from build123d import *

# Parameters (mm, degrees)
DODANIE_WYCI_GNI_CIE1_DEPTH = 180
WYTNIJ_WYCI_GNI_CIE1_DEPTH  = 181.958558792
SZKIC3_R                    = 2.1
DODANIE_WYCI_GNI_CIE2_DEPTH = 3
SFAZOWANIE1_DEPTH           = 3


with BuildPart() as part:
    # Szkic1 → Dodanie-wyciągnięcie1 (new body)
    with BuildSketch(Plane.XY):
        Polygon((0, 0), (10, 0), (10, 3), (3, 3), (3, 6), (11, 6), (11, 7), (7, 15), (6, 15), (6, 9), (3, 9), (3, 15), (0, 15), align=None)
    extrude(amount=DODANIE_WYCI_GNI_CIE1_DEPTH)

    # Szkic2 → Wytnij-wyciągnięcie1 (cut, through all)
    with BuildSketch(Plane(origin=(0, 15, 0), x_dir=(1, 0, 0), z_dir=(0, 1, 0))):
        Polygon((0, -180), (11, -180), (0, -169), align=None)
    extrude(amount=-WYTNIJ_WYCI_GNI_CIE1_DEPTH, mode=Mode.SUBTRACT)

    # Szkic3 → Dodanie-wyciągnięcie2 (add)
    # profile 1 of 2: a face of its own
    with BuildSketch(Plane.ZY):
        with BuildLine():
            Line((25, 20), (25, 11.336506418))
            Line((25, 11.336506418), (35, 11.336506418))
            Line((35, 11.336506418), (35, 20))
            ThreePointArc((35, 20), (30, 25), (25, 20))
        make_face()
        with Locations((30, 20)):
            Circle(SZKIC3_R, mode=Mode.SUBTRACT)
    # profile 2 of 2: a face of its own
    with BuildSketch(Plane.ZY):
        with BuildLine():
            Line((134, 20), (134, 11.336506418))
            Line((134, 11.336506418), (144, 11.336506418))
            Line((144, 11.336506418), (144, 20))
            ThreePointArc((144, 20), (139, 25), (134, 20))
        make_face()
        with Locations((139, 20)):
            Circle(SZKIC3_R, mode=Mode.SUBTRACT)
    extrude(amount=-DODANIE_WYCI_GNI_CIE2_DEPTH)

    # Sfazowanie1: read off the stored shape, not the designer's step
    # Sfazowanie1 outline → Sfazowanie1 (add)
    with BuildSketch(Plane.YZ):
        with BuildLine():
            Line((15, 134), (15, 124.857864376))
            Line((15, 124.857864376), (21.666666667, 134.285954792))
            ThreePointArc((21.666666667, 134.285954792), (20.845509894, 134.072007202), (20, 134))
            Line((20, 134), (15, 134))
        make_face()
        with BuildLine():
            Line((15, 15.857864376), (21.666666667, 25.285954792))
            ThreePointArc((21.666666667, 25.285954792), (20.845509894, 25.072007202), (20, 25))
            Line((20, 25), (15, 25))
            Line((15, 25), (15, 15.857864376))
        make_face()
        with BuildLine():
            Line((21.666666667, 34.714045208), (15, 44.142135624))
            Line((15, 44.142135624), (15, 35))
            Line((15, 35), (20, 35))
            ThreePointArc((20, 35), (20.845509894, 34.927992798), (21.666666667, 34.714045208))
        make_face()
        with BuildLine():
            ThreePointArc((20, 144), (20.845509894, 143.927992798), (21.666666667, 143.714045208))
            Line((21.666666667, 143.714045208), (15, 153.142135624))
            Line((15, 153.142135624), (15, 144))
            Line((15, 144), (20, 144))
        make_face()
    extrude(amount=SFAZOWANIE1_DEPTH)


solid = part.part
The model under review builds one solid part; all positions refer to its coordinate system, in mm. A direction names the side the tool comes from. Give positions to 0.01 mm unless a question says otherwise; leave off trailing zeros. Write each loop counter-clockwise with the first axis right and the second up, starting at its lowest first coordinate (ties: lowest second). Pieces come first, ordered by that corner, then holes.
1. Wall thickness on L1, parallel to Y at x = 5, z = 102; L2, parallel to Y at x = 1.75, z = 30; L3, parallel to X at y = 9.5, z = 31.5: over which ranges is each line inside the solid? List them lowest first.
2. Tool access review of faces 1 (the flat face through (3, 4, 85)), 2 (the flat face through (1.48, 18.38, 39.36)), 3 (the flat face through (6, 12, 86)), 4 (the flat face through (2, 15, 8)), 5 (the flat face through (10, 1, 88)): name each direction out of +Z, -Z, +X, -X, +Y, -Y from which nothing blocks a thin tool from reaching the whole face with its end or side.
3. For P1, Ø1.5, axis at y = 4, z = 78, coming from the +X side; P2, Ø1.5, axis at y = 18, z = 124.5, coming from the -X side; P3, Ø2.5, axis at x = 1, z = 92, coming from the +Y side; P4, Ø8, axis at y = 14, z = 50.5, coming from the +X side, all flat-tipped, find the tip position at first contact; note any pin that passes through.
4. Draft analysis for pull direction Z (two halves, no side actions). For faces 6 (the flat face through (0, 10, 86)), 7 (the flat face through (1.48, 18.38, 148.36)), 8 (the flat face through (4, 8, 0)), 9 (the flat face through (2, 15, 84)), state which applies: +Z half, -Z half, draft (parallel to the pull), parting line (faces both ways), or undercut.
5. Add section C-C, the plane z = 101.5. Write out the cut boundary in (x, y), plus the area to 3 significant figures.
6. Add section A-A, the plane z = 139. Write out the cut boundary in (x, y), plus the area to 3 significant figures.
7. Add section B-B, the plane y = 20. Write out the cut boundary in (x, z).
8. Add section D-D, the plane y = 4.5. Write out the cut boundary in (x, z).
Worked answers:
1. L1: y = 0 to 3, 6 to 9
1. L2: y = 0 to 17.9, 22.1 to 25
1. L3: x = 0 to 3, 6 to 9.75
2. face 1: +Z, -Z, +X
2. face 2: +X, -X, +Y
2. face 3: +Z, -Z, +Y
2. face 4: -Z, +X, -X, +Y
2. face 5: +Z, -Z, +X, -Y
3. P1: stops at x = 3
3. P2: passes through
3. P3: stops at y = 15
3. P4: stops at x = 9.5
4. face 6: draft
4. face 7: +Z half
4. face 8: -Z half
4. face 9: undercut
5. outline: (0, 0) - (10, 0) - (10, 3) - (3, 3) - (3, 6) - (11, 6) - (11, 7) - (7, 15) - (6, 15) - (6, 9) - (3, 9) - (3, 15) - (0, 15) - close
5. area: 104 mm2
6. outline: (0, 0) - (10, 0) - (10, 3) - (3, 3) - (3, 6) - (11, 6) - (11, 7) - (7, 15) - (6, 15) - (6, 9) - (3, 9) - (3, 17.9) - (0, 17.9) - close; (0, 22.1) - (3, 22.1) - (3, 25) - (0, 25) - close
6. area: 121 mm2
7. outline: (0, 22.93) - (3, 22.93) - (3, 27.9) - (0, 27.9) - close; (0, 32.1) - (3, 32.1) - (3, 37.07) - (0, 37.07) - close; (0, 131.93) - (3, 131.93) - (3, 136.9) - (0, 136.9) - close; (0, 141.1) - (3, 141.1) - (3, 146.07) - (0, 146.07) - close
8. outline: (0, 0) - (3, 0) - (3, 172) - (0, 169) - close
